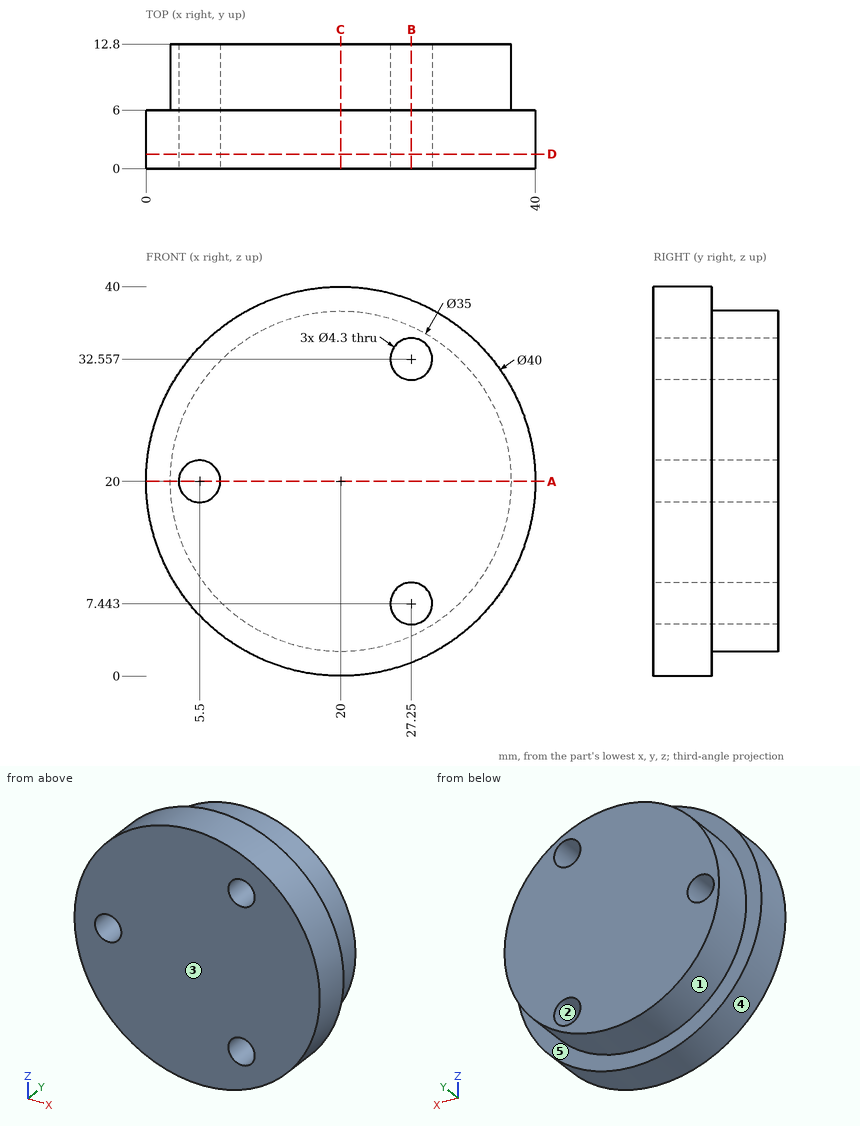
Job drawing, mm, ordinate dimensions from the low corner. One solid piece. A direction names the side the tool comes from. Coordinates: 2 decimals unless noted, no trailing zeros. Loops run counter-clockwise (first coordinate to the right, second up) from the corner with the lowest first, then second, coordinate; pieces in that order, holes last. Notation, with made-up numbers: (60, -10) - (116, -10) arc R16 ccw to (116, 4) - close; hole circle Ø10 at (2.5, 8). An arc over 180 degrees is marked (long way). Answer as a JSON object with one key per item and string values. Group by question number.
(1) Tool access for the marked faces 4 and 5: list every direction of +Z, -Z, +X, -X, +Y, -Y with a clear straight run to the whole face (end or side of a thin tool).
(2) Flat gauge pins, fed straight in: pin 1 (1 mm diameter, centred on y = 11.5, z = 32.5, fed in from -X); pin 2 (5 mm diameter, centred on y = 11, z = 28.5, fed in from -X); pin 3 (2 mm diameter, centred on x = 36, y = 8.5, fed in from -Z) (1 decimal); pin 4 (4 mm diameter, centred on x = 15.5, z = 16, fed in from -Y). Where does each tip first touch, or does it go through?
(3) Cut at B-B (x = 27.25). Give the cut face in (y, z).
(4) Cut at C-C (x = 20). Give the cut face in (y, z), then the cut area to 3 significant figures.
(5) Two-plate mould, pull along X, no slides. Class the marked faces 1, 2 and 3: released by +X, released by -X, zero draft, split by the parting line, or undercut.
(6) Cut at A-A (z = 20). Give the cut face in (x, y), then the cut area to 3 significant figures.
(7) Probe line 1 along Z through (x, y) = (27.25, 10); line 2 along X through (y, z) = (9.75, 20); line 3 along Z through (x, y) = (28.5, 8.75) (1 decimal). List the from-to ranges inside material, lowest first.
(8) Cut at D-D (y = 1.5). Give the cut face in (x, z).
Geometry says:
{
 "1": {"face 4": "+Y, -Y", "face 5": "+Y"},
 "2": {"pin 1": "stops at x = 7.26", "pin 2": "stops at x = 3.56", "pin 3": "stops at z = 11", "pin 4": "stops at y = 0"},
 "3": {"outline": "(0, 1.36) - (6, 1.36) - (6, 4.07) - (12.8, 4.07) - (12.8, 5.29) - (0, 5.29) - close; (0, 9.59) - (12.8, 9.59) - (12.8, 30.41) - (0, 30.41) - close; (0, 34.71) - (12.8, 34.71) - (12.8, 35.93) - (6, 35.93) - (6, 38.64) - (0, 38.64) - close"},
 "4": {"outline": "(0, 0) - (6, 0) - (6, 2.5) - (12.8, 2.5) - (12.8, 37.5) - (6, 37.5) - (6, 40) - (0, 40) - close", "area": "478 mm^2"},
 "5": {"face 1": "split by the parting line", "face 2": "undercut", "face 3": "zero draft"},
 "6": {"outline": "(0, 0) - (3.35, 0) - (3.35, 12.8) - (2.5, 12.8) - (2.5, 6) - (0, 6) - close; (7.65, 0) - (40, 0) - (40, 6) - (37.5, 6) - (37.5, 12.8) - (7.65, 12.8) - close", "area": "423 mm^2"},
 "7": {"line 1": "z = 4.07 to 5.29, 9.59 to 30.41, 34.71 to 35.93", "line 2": "x = 2.5 to 3.35, 7.65 to 37.5", "line 3": "z = 4.7 to 5.7, 9.2 to 30.8, 34.3 to 35.3"},
 "8": {"outline": "circle Ø40 at (20, 20); hole circle Ø4.3 at (5.5, 20); hole circle Ø4.3 at (27.25, 7.44); hole circle Ø4.3 at (27.25, 32.56)"}
}
